Autodesk Inventor part; units mm, degrees
ref_plane "Work Plane1" through (0, -77.0641, 0) normal (0, 1, 0) x (-1, 0, 0)
ref_plane "Work Plane3" through (0, 0, -34.98) normal (0, 0, 1) x (1, 0, 0)
ref_plane "YZ Plane" through (0, 0, 0) normal (1, 0, 0) x (0, 1, 0)
sketch "Sketch2" plane through (0, 0, 0) normal (0, 0, 1) x (1, 0, 0)
  line L0 (0, 0) -> (0, 152.4)
  line L1 (30.98, 3.1589) -> (30.98, 101.6)
  arc A0 (107.18, 92.6021) -> (32.1988, 2.9089) centre (218.9996, -77.0641) ccw
  arc A1 (30.98, 3.1589) -> (32.1988, 2.9089) centre (31.615, 3.1589) ccw
  line L2 (30.98, 101.6) -> (30.98, 127)
  arc A2 (107.18, 92.6021) -> (30.98, 127) centre (30.98, 25.4) ccw
  line L3 (30.98, 127) -> (25.9, 127)
  line L4 (31.98, 125.995) -> (31.98, 101.6)
  line L5 (31.98, 101.6) -> (31.98, 4.9195)
  arc A3 (105.6655, 92.7976) -> (31.98, 4.9195) centre (218.9996, -77.0641) ccw
  arc A4 (105.6655, 92.7976) -> (31.98, 125.995) centre (30.98, 25.4) ccw
  point P0 (30.98, 0)
  point P1 (43.68, 0)
  point P2 (119.8707, 100.316)
  dimension "d0" = 30.98
  dimension "d1" = 101.6
  dimension "d2" = 152.4
  dimension "d76" = 88.9
  dimension "d77" = 203.2
  dimension "d80" = 0.635
  dimension "d91" = 25.4
  dimension "d92" = 101.6
  dimension "d93" = 76.2
  dimension "d94" = 5.08
  dimension "d95" = 0
  dimension "d96" = 1
revolve "Revolution1" add sketch "Sketch2" angle 360 about axis through (0, 0, 0) along (0, 1, 0)
ref_plane "Work Plane1" through (0, -77.0641, 0) normal (0, 1, 0) x (-1, 0, 0)
sketch "Sketch4" plane through (0, -77.0641, 0) normal (0, 1, 0) x (-1, 0, 0)
  circle A0 centre (0, 88.9) radius 3
  line L0 (0, 0) -> (0, 115.8951)
  dimension "d19" = 6
  dimension "d20" = 88.9
extrude "Extrusion1" cut sketch "Sketch4" along normal blind 174.625
pattern_circular "Circular Pattern1" count 3 over 360 about axis through (0, 65.0794, 0) along (0, 1, 0) of "Extrusion1"
sketch "Sketch11" plane through (0, 0, 0) normal (0, 1, 0) x (-1, 0, 0)
  circle A0 centre (0, 0) radius 34.98
  circle A1 centre (0, 0) radius 30.98
  circle A2 centre (0, 0) radius 30.98
  dimension "d83" = 0
  dimension "d84" = 4
extrude "Extrusion7" add sketch "Sketch11" along normal blind 12.7 and the other way blind 8.89
ref_plane "Work Plane3" through (0, 0, -34.98) normal (0, 0, 1) x (1, 0, 0)
sketch "Sketch12" plane through (0, 0, -34.98) normal (0, 0, 1) x (1, 0, 0)
  line L0 (4.54, 0) -> (2.54, 0)
  line L1 (2.54, 0) -> (2.54, -8.89)
  line L2 (2.54, -8.89) -> (4.54, -8.89)
  line L3 (4.54, -8.89) -> (4.54, 0)
  line L4 (-2.54, 0) -> (-4.54, 0)
  line L5 (-4.54, 0) -> (-4.54, -8.89)
  line L6 (-4.54, -8.89) -> (-2.54, -8.89)
  line L7 (-2.54, -8.89) -> (-2.54, 0)
  line L8 (0, -8.89) -> (0, 0)
  line L9 (-34.98, -8.89) -> (34.98, -8.89)
  dimension "d56" = 8.89
  dimension "d57" = 2
  dimension "d58" = 2.54
  dimension "d85" = 0
extrude "Extrusion8" add sketch "Sketch12" along normal blind 1.27 and the other way blind 8.89
sketch "Sketch13" plane through (0, 0, -34.98) normal (0, 0, 1) x (1, 0, 0)
  line L0 (2.54, 0) -> (2.54, -8.89)
  line L1 (-2.54, -8.89) -> (2.54, -8.89)
  line L2 (2.54, 0) -> (-2.54, 0)
  line L3 (-2.54, 0) -> (-2.54, -8.89)
  line L4 (-2.54, -8.89) -> (2.54, -8.89)
  line L5 (2.54, -8.89) -> (2.54, 0)
  point P0 (0, 0)
extrude "Extrusion9" cut sketch "Sketch13" along normal up to surface
sketch "Sketch15" plane through (0, 0, -43.87) normal (0, 0, -1) x (-1, 0, 0)
  line L0 (2.54, -8.89) -> (2.54, 0)
  line L1 (34.98, -8.89) -> (34.98, 9.1161)
  line L2 (2.54, 0) -> (34.98, 0)
  line L3 (34.98, 0) -> (34.98, -2)
  line L4 (34.98, -2) -> (2.54, -2)
  line L5 (2.54, -2) -> (2.54, 0)
  point P0 (0, 0)
  dimension "d89" = 2
extrude "Extrusion10" cut sketch "Sketch15" against normal blind 63.5
sketch "Sketch16" plane through (-4.54, 0, -43.87) normal (-1, 0, 0) x (0, 0, 1)
  line L0 (2.54, -8.89) -> (2.54, 0)
  line L1 (0, -8.89) -> (0, 0)
  circle A0 centre (2.54, -3.81) radius 1.27
  circle A1 centre (2.54, -6.985) radius 1.27
  line L2 (9.1859, 0) -> (0, 0)
  line L3 (0, -8.89) -> (9.1859, -8.89)
  point P0 (43.87, 0)
  dimension "d68" = 2.54
  dimension "d69" = 2.54
  dimension "d70" = 2.54
  dimension "d71" = 3.81
  dimension "d90" = 1.905
extrude "Extrusion11" cut sketch "Sketch16" against normal up to surface (9.08 mm away) contours A1 L0 | L0 A1 | A0 L0 | L0 A0
properties part number "Water Sensor Bouy 3_3DPrint"
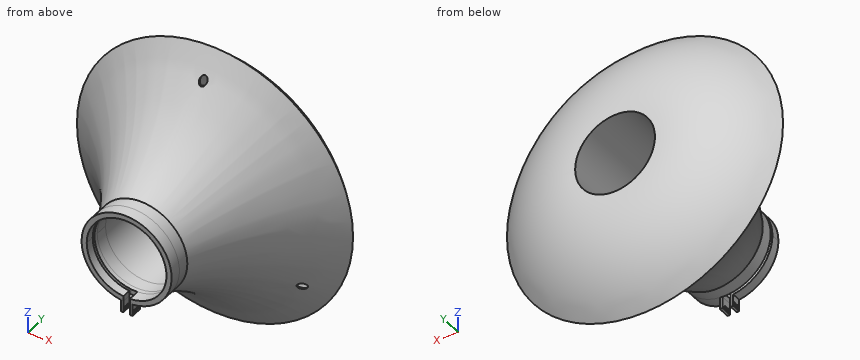
Input: part model. Units: mm. Frame: model coordinates. Coordinates: 2 decimals unless noted, no trailing zeros. Loops run counter-clockwise (first coordinate to the right, second up) from the corner with the lowest first, then second, coordinate; pieces in that order, holes last. Notation, with made-up numbers: M 50,74 L 87,74 A16 ccw 87,96 Z; hole C 54,23.5 d11. An arc over 180 degrees is marked long. One line per item, written item: value.
(1) Line query: line 1 along Y through (x, z) = (-19, -28); line 2 along Z through (x, y) = (17, 75); line 3 along Z through (x, y) = (-28, 91.5). Output: solid intervals per line, ascending. Write a range as from..to.
Filled in:
line 1: -8.89..-2, 0..12.7, 125.96..126.96
line 2: -82.48..-80.95, -27.09..-25.9, 25.9..27.09, 80.95..82.48
line 3: -101.74..-99.89, -15.45..-13.26, 13.26..15.45, 99.89..101.74
(2) Section B-B (z = -14). Give the number of separate pieces and of enclosed holes in the cut face, and give its area (3 significant figures).
Filled in:
separate pieces: 3
enclosed holes: 2
area: 838 mm^2
(3) Section A-A (y = 28). Output: boundary loops of the cut face in (x, z).
Filled in:
outline: C 0,0 d90.14; C 0,0 d63.96; hole C 0,0 d87.8; hole C 0,0 d61.96
(4) Pin query (flat end, axial travel): pin 1 (2.5 mm diameter, centred on y = -5, z = -41, fed in from -X); pin 2 (12 mm diameter, centred on y = 53, z = 35, fed in from -X); pin 3 (3 mm diameter, centred on x = 1.5, z = 37.5, fed in from -Y); pin 4 (21 mm diameter, centred on x = 7, z = -9, fed in from +Y). Return the tip coordinate at first contact, or that it passes through.
Filled in:
pin 1: x = -4.54
pin 2: x = -59.28
pin 3: y = 11.32
pin 4: through
